Autodesk Inventor part; units mm, degrees
ref_plane "YZ Plane" through (0, 0, 0) normal (1, 0, 0) x (0, 1, 0)
ref_plane "XZ Plane" through (0, 0, 0) normal (0, 1, 0) x (-1, 0, 0)
ref_plane "XY Plane" through (0, 0, 0) normal (0, 0, 1) x (1, 0, 0)
sketch "Sketch1" plane through (0, 0, 0) normal (1, 0, 0) x (0, 1, 0)
  line L0 (0, 0) -> (45, 0)
  line L1 (45, 0) -> (45, -11)
  line L2 (45, -11) -> (0, -11)
  line L3 (0, -11) -> (0, 0)
  line L4 (0, -11) -> (45, -11)
  line L5 (45, -11) -> (45, -2)
  line L6 (45, -2) -> (0, -2)
  line L7 (0, -2) -> (0, -11)
  line L8 (45, -11) -> (47, -11)
  line L9 (47, -11) -> (47, -6)
  line L10 (47, -6) -> (45, -6)
  line L11 (45, -6) -> (45, -11)
  point P0 (0, -2)
  dimension "d1" = 11
  dimension "d2" = 45
  dimension "d39" = 2
  dimension "d40" = 2
  dimension "d41" = 5
revolve "Revolution1" add sketch "Sketch1" angle 360 about axis through (0, 0, 0) along (0, 1, 0) contours L6 L1 L2 L3 | L10 L9 L8 L1
sketch "Sketch2" plane through (0, 0, 0) normal (1, 0, 0) x (0, 1, 0)
  circle A0 centre (32, 0) radius 2
  line L0 (45, 6) -> (45, -6)
  point P0 (0, 0)
  dimension "d8" = 4
  dimension "d42" = 13
extrude "Extrusion1" cut sketch "Sketch2" along normal through all both and the other way through all
sketch "Sketch3" plane through (0, 0, 0) normal (0, 0, 1) x (1, 0, 0)
  circle A0 centre (0, 32) radius 2
  line L0 (-6, 45) -> (6, 45)
  point P0 (0, 0)
  dimension "d13" = 4
  dimension "d43" = 13
extrude "Extrusion2" cut sketch "Sketch3" against normal through all both and the other way through all
properties part number "shaft"
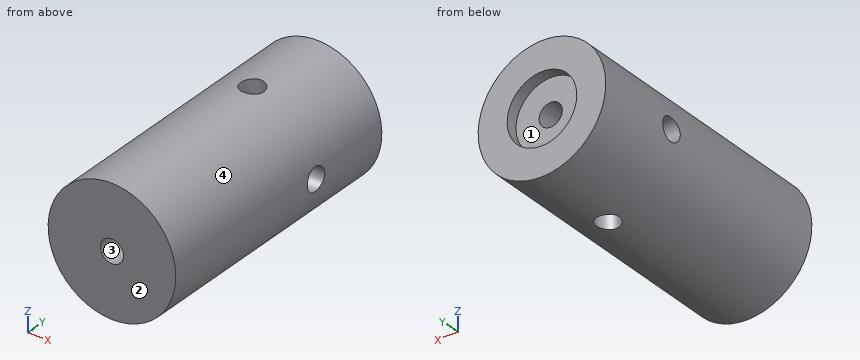
Verification items for the finished model (mm, model axes). Face numbers are marked on the shaded views. Round coordinates to 2 decimals unless told otherwise and drop trailing zeros. Order: outer loops, then holes, each group sorted by start corner. A loop starts at its lowest first (then second) coordinate and runs counter-clockwise, first axis right, second up.
1) Cross-section at B-B, the plane x = 0. Record the cut outline in (y, z).
Geometry says:
outline: (0, -11) - (30, -11) - (30, -2) - (0, -2) - close; (0, 2) - (30, 2) - (30, 11) - (0, 11) - close; (34, -11) - (47, -11) - (47, -6) - (45, -6) - (45, -2) - (34, -2) - close; (34, 2) - (45, 2) - (45, 6) - (47, 6) - (47, 11) - (34, 11) - close
2) Material ranges on line 1 (Z direction, x = 0, y = 46.15); line 2 (Z direction, x = 0, y = 23); line 3 (Y direction, x = 7.5, z = 0), recorded low to high.
Geometry says:
line 1: z = -11 to -6, 6 to 11
line 2: z = -11 to -2, 2 to 11
line 3: y = 0 to 30, 34 to 47
3) Cross-section at A-A, the plane z = 0. Record the cut outline in (x, y), plus the area to 3 significant figures.
Geometry says:
outline: (-11, 0) - (-2, 0) - (-2, 30) - (-11, 30) - close; (-11, 34) - (-2, 34) - (-2, 45) - (-6, 45) - (-6, 47) - (-11, 47) - close; (2, 0) - (11, 0) - (11, 30) - (2, 30) - close; (2, 34) - (11, 34) - (11, 47) - (6, 47) - (6, 45) - (2, 45) - close
area: 758 mm2
4) Draft check along Z on the marked faces 1, 2, 3 and 4. Enter one of: +Z half, -Z half, draft (parallel to the pull), parting line (faces both ways), or undercut.
Geometry says:
face 1: undercut
face 2: draft
face 3: undercut
face 4: parting line
5) Cross-section at D-D, the plane z = -6.5. Record the cut outline in (x, y), plus the area to 3 significant figures.
Geometry says:
outline: (-8.87, 0) - (8.87, 0) - (8.87, 47) - (-8.87, 47) - close; hole circle Ø4 at (0, 32)
area: 822 mm2
6) Cross-section at C-C, the plane y = 25. Record the cut outline in (x, z), plus the area to 3 significant figures.
Geometry says:
outline: circle Ø22 at (0, 0); hole circle Ø4 at (0, 0)
area: 368 mm2
7) Depth check by flat-ended pin: pin 1 (6.5 mm diameter, centred on x = 0, z = 0, fed in from +Y); pin 2 (6 mm diameter, centred on y = 24, z = 3.5, fed in from -X); pin 3 (1.5 mm diameter, centred on x = 8.5, y = 7.5, fed in from -Z). Enter the tip coordinate at first touch or a pass-through.
Geometry says:
pin 1: stops at y = 45
pin 2: stops at x = -10.99
pin 3: stops at z = -7.81
